```python
from build123d import *

# Parameters (mm, degrees)
SKETCH1_R               = 4.7625
BOSS_EXTRUDE1_DEPTH     = 25.4
SKETCH2_RX              = 4.7625
SKETCH2_RY              = 1.232625702
SKETCH2_RX_2            = 9.362827468
SKETCH2_RY_2            = 1.051298719
CUT_EXTRUDE1_DEPTH      = 27.277800755
CUT_EXTRUDE1_DEPTH_BACK = 27.277800755


with BuildPart() as part:
    # Sketch1 → Boss-Extrude1 (new body)
    with BuildSketch(Plane.XY):
        Circle(SKETCH1_R)
    extrude(amount=BOSS_EXTRUDE1_DEPTH)

    # Sketch2 → Cut-Extrude1 (cut, two sides)
    with BuildSketch(Plane(origin=(0, 0, 0), x_dir=(0, 1, 0), z_dir=(-0.9659258262890691, 0, -0.2588190451025179))) as cut_extrude1_sk:
        with Locations(Location((0, 0), (0, 0, 180))):
            Ellipse(SKETCH2_RX, SKETCH2_RY)
        with Locations((0, -2.93730779)):
            Ellipse(SKETCH2_RX_2, SKETCH2_RY_2)
    extrude(amount=CUT_EXTRUDE1_DEPTH, mode=Mode.SUBTRACT)
    extrude(cut_extrude1_sk.sketch, amount=-CUT_EXTRUDE1_DEPTH_BACK, mode=Mode.SUBTRACT)


with BuildPart() as cut_extrude1_kept_piece:
    # of the separate pieces the step leaves, the one the design keeps (cut_extrude1_pieces_kept)
    add(part.part.solids().sort_by_distance((-0.996279445, 4.657127174, 3.718165509))[0])


solid = cut_extrude1_kept_piece.part
```
Here's how the part is built. I have some questions about the finished solid (model axes, mm). Coordinates: 2 decimals unless noted, no trailing zeros. Loops run counter-clockwise (first coordinate to the right, second up) from the corner with the lowest first, then second, coordinate; pieces in that order, holes last. Notation, with made-up numbers: (-17.5, 46.5) -> (15.5, 46.5) arc R19 ccw to (15.5, 81.5) -> close; hole circle Ø2 at (16, 63). An arc over 180 degrees is marked (long way). Return JSON: item names as keys, results as strings.
1) Will these pins go through, and if not, where does the flat tip stop? pin 1 (3 mm diameter, centred on y = -3.5, z = 14.5, fed in from -X); pin 2 (1.5 mm diameter, centred on y = 1, z = 8.5, fed in from -X); pin 3 (1 mm diameter, centred on x = -2, z = 5.5, fed in from -Y).
Results below:
{"pin 1": "x = -4.32", "pin 2": "x = -4.76", "pin 3": "y = -4.52"}
2) I need wall thicknesses on line 1 (Y direction, x = -1, z = 18.5); line 2 (Y direction, x = 3.5, z = 23.5); line 3 (X direction, y = 3.75, z = 23.75). Which ranges of each line are inside material? Lowest first, please. Write a range as from..to.
Results below:
{"line 1": "-4.66..4.66", "line 2": "-3.23..3.23", "line 3": "-2.94..2.94"}
3) If we section it at A-A, the plane z = 13: Write out the boundary of the cut face in (x, y) (1 decimal).
Results below:
{"outline": "circle Ø9.5 at (0, 0)"}
